Source: CAD feature listing. Evaluate the final solid. Frame: model axes, mm. Round coordinates to 2 decimals unless told otherwise and drop trailing zeros. Loops run counter-clockwise (first coordinate to the right, second up) from the corner with the lowest first, then second, coordinate; pieces in that order, holes last.
(1) Section C-C, the plane x = 2.54. Return the cut outline in (y, z).
(2) Section A-A, the plane z = 6.35. Return the cut outline in (x, y).
(3) Material intervals for probe 1 along X at (y, z) = (-1.75, 6.35); probe 2 along Y at (x, z) = (-7.62, 9); probe 3 along Z at (x, y) = (7.62, 1), sorted ascending.
(4) Section B-B, the plane y = 0. Return the cut outline in (x, z).
(5) Section D-D, the plane z = 11.25. Return the cut outline in (x, y).
(6) First-contact query: pin 1 Ø3 at (x, y) = (2, -2) entering from -Z. Flat tip, straight axial feed; report the tip coordinate or a pass-through.
(7) Mould query, pull axis Z, two halves, no side actions, for faces 1 (the flat face through (0, 0, 12.7)), 2 (the cylindrical face through (-2.25, -0.09, 7.67)), 3 (the flat face through (12.7, 0, 6)). Classes: pulls with the +Z half, pulls with the -Z half, needs draft (parallel to the pull), parting line crosses it, or undercut.
```python
from build123d import *

# Parameters (mm, degrees)
SKETCH1_W                 = 25.4
SKETCH1_H                 = 12.7
BOSS_EXTRUDE1_DEPTH       = 12.7
TAP_DRILL_FOR_6_32_TAP1_D = 2.7051
TAP_DRILL_FOR_6_32_TAP2_D = 2.7051


with BuildPart() as part:
    # Sketch1 → Boss-Extrude1 (new body)
    with BuildSketch(Plane.XY):
        Rectangle(SKETCH1_W, SKETCH1_H)
    extrude(amount=BOSS_EXTRUDE1_DEPTH)

    # Tap Drill for #6-32 Tap1 (through all)
    with Locations(Plane(origin=(0, 6.35, 0), x_dir=(1, 0, 0), z_dir=(0, 1, 0))):
        with Locations((-2.54, -6.35), (7.62, -6.35)):
            Hole(TAP_DRILL_FOR_6_32_TAP1_D / 2)

    # Tap Drill for #6-32 Tap2 (through all)
    with Locations(Plane.XY.offset(12.7)):
        with Locations((-7.62, 0), (2.54, 0)):
            Hole(TAP_DRILL_FOR_6_32_TAP2_D / 2)


solid = part.part
```
Output values:
1. outline: (-6.35, 0) - (-1.35, 0) - (-1.35, 12.7) - (-6.35, 12.7) - close; (1.35, 0) - (6.35, 0) - (6.35, 12.7) - (1.35, 12.7) - close
2. outline: (-12.7, -6.35) - (-3.89, -6.35) - (-3.89, 6.35) - (-12.7, 6.35) - close; (-1.19, -6.35) - (6.27, -6.35) - (6.27, 6.35) - (-1.19, 6.35) - close; (8.97, -6.35) - (12.7, -6.35) - (12.7, 6.35) - (8.97, 6.35) - close; hole circle Ø2.71 at (-7.62, 0); hole circle Ø2.71 at (2.54, 0)
3. probe 1: x = -12.7 to -3.89, -1.19 to 6.27, 8.97 to 12.7
3. probe 2: y = -6.35 to -1.35, 1.35 to 6.35
3. probe 3: z = 0 to 5, 7.7 to 12.7
4. outline: (-12.7, 0) - (-8.97, 0) - (-8.97, 12.7) - (-12.7, 12.7) - close; (-6.27, 0) - (1.19, 0) - (1.19, 12.7) - (-6.27, 12.7) - close; (3.89, 0) - (12.7, 0) - (12.7, 12.7) - (3.89, 12.7) - close; hole circle Ø2.71 at (-2.54, 6.35); hole circle Ø2.71 at (7.62, 6.35)
5. outline: (-12.7, -6.35) - (12.7, -6.35) - (12.7, 6.35) - (-12.7, 6.35) - close; hole circle Ø2.71 at (-7.62, 0); hole circle Ø2.71 at (2.54, 0)
6. pin 1: stops at z = 0
7. face 1: pulls with the +Z half
7. face 2: undercut
7. face 3: needs draft
